```python
from build123d import *

# Parameters (mm, degrees)
BOSS_EXTRUDE1_DEPTH = 18
SKETCH2_R           = 4.5
CUT_EXTRUDE1_DEPTH  = 41
SKETCH3_R           = 4.5
CUT_EXTRUDE2_DEPTH  = 41


with BuildPart() as part:
    # Sketch1 → Boss-Extrude1 (new body, symmetric)
    with BuildSketch(Plane.XY):
        with BuildLine():
            Line((0, 0), (0, 40))
            ThreePointArc((0, 40), (4.242640687, 38.242640687), (6, 34))
            Line((6, 34), (6, 12))
            ThreePointArc((6, 12), (7.757359313, 7.757359313), (12, 6))
            Line((12, 6), (34, 6))
            ThreePointArc((34, 6), (38.242640687, 4.242640687), (40, 0))
            Line((40, 0), (0, 0))
        make_face()
    extrude(amount=BOSS_EXTRUDE1_DEPTH, both=True)

    # Sketch2 → Cut-Extrude1 (cut, through all)
    with BuildSketch(Plane(origin=(0, 0, 0), x_dir=(1, 0, 0), z_dir=(0, 1, 0))):
        with Locations((20, 0)):
            Circle(SKETCH2_R)
    extrude(amount=CUT_EXTRUDE1_DEPTH, mode=Mode.SUBTRACT)

    # Sketch3 → Cut-Extrude2 (cut, through all)
    with BuildSketch(Plane(origin=(0, 0, 0), x_dir=(0, 0, -1), z_dir=(1, 0, 0))):
        with Locations((0, 20)):
            Circle(SKETCH3_R)
    extrude(amount=CUT_EXTRUDE2_DEPTH, mode=Mode.SUBTRACT)


solid = part.part
```
Here's how the part is built. I have some questions about the finished solid (model axes, mm). A direction names the side the tool comes from. Coordinates: 2 decimals unless noted, no trailing zeros. Write each loop counter-clockwise with the first axis right and the second up, starting at its lowest first coordinate (ties: lowest second). Pieces come first, ordered by that corner, then holes. Notation, with made-up numbers: M 24,65.5 L 83,65.5 A18 ccw 83,87.5 Z; hole C 76,-27 d4. An arc over 180 degrees is marked long. Answer as CSV lines item,"result". Start each with the question number.
Q1. Suppose I cut it at C-C, the plane z = 11. List the corners of the cut face in (x, y) for me, then the cut area to 3 significant figures.
Q2. I need wall thicknesses on probe 1 along Z at (x, y) = (2, 20); probe 2 along Y at (x, z) = (12.5, 11); probe 3 along X at (y, z) = (1.7, 0). Which ranges of each line are inside material? Lowest first, please. Write a range as [from, to].
Q3. Will these pins go through, and if not, where does the flat tip stop? pin 1 Ø5 at (x, z) = (30.5, 5) entering from +Y; pin 2 Ø7 at (y, z) = (20, 0) entering from +X.
Q4. For faces 4 (the flat face through (0, 15, 0)), 5 (the flat face through (25, 6, 0)), which set-ups out of +Z, -Z, +X, -X, +Y, -Y let a thin tool reach every point of the face, with its end or its side?
Q5. Suppose I cut it at D-D, the plane z = 2.5. List the corners of the cut face in (x, y) for me, then the cut area to 3 significant figures.
Q6. Suppose I cut it at A-A, the plane y = 20. List the corners of the cut face in (x, z) for me.
Q7. If we mould it in two halves opening along Z, with no side actions, what happens to faces 1 (the cylindrical face through (15.504, 2.958, -0.198)), 2 (the cylindrical face through (4.196, 38.289, 0.252)), 3 (the flat face through (8, 7, -18))? For each: pulls with the +Z half, pulls with the -Z half, needs draft (parallel to the pull), parting line crosses it, or undercut.
Entries:
1,outline,"M 0,0 L 40,0 A6 ccw 34,6 L 12,6 A6 cw 6,12 L 6,34 A6 ccw 0,40 Z"
1,area,"436 mm²"
2,probe 1,"z = [-18, -4.5], [4.5, 18]"
2,probe 2,"y = [0, 6]"
2,probe 3,"x = [0, 15.5], [24.5, 39.75]"
3,pin 1,"stops at y = 6"
3,pin 2,"passes through"
4,face 4,"+Z, -Z, -X, +Y, -Y"
4,face 5,"+Z, -Z, +X, +Y"
5,outline,"M 0,0 L 16.26,0 L 16.26,6 L 12,6 A6 cw 6,12 L 6,16.26 L 0,16.26 Z; M 0,23.74 L 6,23.74 L 6,34 A6 ccw 0,40 Z; M 23.74,0 L 40,0 A6 ccw 34,6 L 23.74,6 Z"
5,area,"346 mm²"
6,outline,"M 0,-18 L 6,-18 L 6,-4.5 L 0,-4.5 Z; M 0,4.5 L 6,4.5 L 6,18 L 0,18 Z"
7,face 1,"undercut"
7,face 2,"needs draft"
7,face 3,"pulls with the -Z half"
